from build123d import *

# Parameters (mm, degrees)
F1_DEPTH = 45
F2_DEPTH = 450


# Not quite as in the source:
# - a feature names something its author has since deleted; it is built from what else it names


with BuildPart() as f1:
    # F0 (on Right) → F1 (new body, symmetric)
    with BuildSketch(Plane.YZ):
        with BuildLine():
            ThreePointArc((161.2936216865, 313.43359361), (-300.9254489442, -183.5759357262), (352.5, 0))
            ThreePointArc((352.5, 0), (312.7518796274, 162.6115364588), (202.4715643149, 288.5507158956))
            ThreePointArc((202.4715643149, 288.5507158956), (182.3076165098, 301.6955136599), (161.2936216865, 313.43359361))
        make_face()
        with BuildLine():
            ThreePointArc((161.2936216865, 313.43359361), (182.3076165098, 301.6955136599), (202.4715643149, 288.5507158956))
            Line((202.4715643149, 288.5507158956), (287.6534110047, 454.0802144534))
            Line((287.6534110047, 454.0802144534), (255.5, 496.5))
            Line((255.5, 496.5), (161.2936216865, 313.43359361))
        make_face()
        Polygon((255.5, 496.5), (287.6534110047, 454.0802144534), (595.193856999, 48.3441087551), (1115.193856999, 48.3441087551), (1115.193856999, 259.8511291536), (1115.193856999, 330.4220543775), (1115.193856999, 612.5), (385.6319234642, 612.5), (315.193856999, 612.5), align=None)
        Polygon((495.5619335347, 963), (315.193856999, 612.5), (385.6319234642, 612.5), (566, 963), align=None)
        Polygon((456, 963), (495.5619335347, 963), (566, 963), (566, 1023), (456, 1023), align=None)
        with BuildLine():
            Line((1115.193856999, 330.4220543775), (1115.193856999, 259.8511291536))
            Line((1115.193856999, 259.8511291536), (1195.3817888304, 179.9804793552))
            ThreePointArc((1195.3817888304, 179.9804793552), (1210.9786128275, 199.6313048689), (1228.0043825139, 218.0578897059))
            Line((1228.0043825139, 218.0578897059), (1115.193856999, 330.4220543775))
        make_face()
        with BuildLine():
            ThreePointArc((1228.0043825139, 218.0578897059), (1210.9786128275, 199.6313048689), (1195.3817888304, 179.9804793552))
            ThreePointArc((1195.3817888304, 179.9804793552), (1360.8295666617, -335.8659636043), (1799.5, -18))
            ThreePointArc((1799.5, -18), (1592.7012450035, 291.1644255482), (1228.0043825139, 218.0578897059))
        make_face()
    extrude(amount=F1_DEPTH, both=True)

    # F0 (on Right) → F2 (join, symmetric)
    with BuildSketch(Plane.YZ):
        Polygon((456, 963), (495.5619335347, 963), (566, 963), (566, 1023), (456, 1023), align=None)
    extrude(amount=F2_DEPTH, both=True)


solid = f1.part
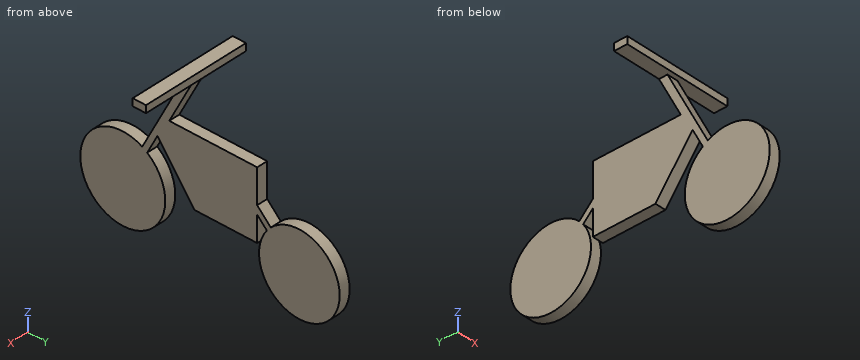
Check sheet for the modelled part. Datum: model origin and axes. Units: mm. Round coordinates to 2 decimals unless told otherwise and drop trailing zeros. Write each loop counter-clockwise with the first axis right and the second up, starting at its lowest first coordinate (ties: lowest second). Pieces come first, ordered by that corner, then holes. Notation, with made-up numbers: (88, 37) - (124, 37) arc R11 cw to (124, 56) - close; hole circle Ø4 at (2, 61.5). An arc over 180 degrees is marked (long way). Return JSON: item names as keys, results as strings.
Q1. Cross-section at B-B (z = 121). Record the boundary of the cut face in (x, y), then the cut area to 3 significant figures.
Returned:
{"outline": "(-45, -331.08) - (45, -331.08) - (45, 331.08) - (-45, 331.08) - close; (-45, 540.12) - (45, 540.12) - (45, 1115.19) - (-45, 1115.19) - close; (-45, 1160.75) - (45, 1160.75) - (45, 1769.25) - (-45, 1769.25) - close", "area": "166,000 mm²"}
Q2. Cross-section at A-A (z = -56). Record the boundary of the cut face in (x, y).
Returned:
{"outline": "(-45, -348.02) - (45, -348.02) - (45, 348.02) - (-45, 348.02) - close; (-45, 1132.67) - (45, 1132.67) - (45, 1797.33) - (-45, 1797.33) - close"}
Q3. Cross-section at C-C (y = 0). Record the boundary of the cut face in (x, z).
Returned:
{"outline": "(-45, -352.5) - (45, -352.5) - (45, 352.5) - (-45, 352.5) - close"}
Q4. Scan lines: L1, parallel to X at y = 669, z = 593; L2, parallel to Y at x = 17.5, z = 786. Record each from-to range of solid material in increasing order. Write a range as from..to.
Returned:
{"L1": "x = -45..45", "L2": "y = 404.48..474.92"}
Q5. Cross-section at D-D (x = -90). Record the boundary of the cut face in (y, z), then the cut area to 3 significant figures.
Returned:
{"outline": "(456, 963) - (566, 963) - (566, 1023) - (456, 1023) - close", "area": "6,600 mm²"}
Q6. Depth check by flat-ended pin: P1, Ø3, axis at y = 510, z = 399, coming from the -X side; P2, Ø10, axis at y = 709.5, z = 553.5, coming from the +X side; P3, Ø2, axis at x = -5.5, y = 656, coming from the -Z side. Enter the tip coordinate at first touch or a pass-through.
Returned:
{"P1": "stops at x = -45", "P2": "stops at x = 45", "P3": "stops at z = 48.34"}
